Autodesk Inventor part; units mm, degrees
ref_plane "YZ Plane" through (0, 0, 0) normal (1, 0, 0) x (0, 1, 0)
ref_plane "XZ Plane" through (0, 0, 0) normal (0, 1, 0) x (-1, 0, 0)
ref_plane "XY Plane" through (0, 0, 0) normal (0, 0, 1) x (1, 0, 0)
sketch "Sketch1" plane through (0, 0, 0) normal (0, 1, 0) x (-1, 0, 0)
  line L0 (-35, 35) -> (35, 35)
  line L1 (35, 35) -> (35, -35)
  line L2 (35, -35) -> (-35, -35)
  line L3 (-35, -35) -> (-35, 35)
  line L4 (-35, 35) -> (35, -35) construction
  line L5 (35, 35) -> (-35, -35) construction
  point P0 (0, 0)
  dimension "d0" = 70
  dimension "d1" = 70
extrude "Extrusion1" add sketch "Sketch1" along normal blind 1
sketch "Sketch2" plane through (0, 1, 0) normal (0, 1, 0) x (1, 0, 0)
  line L0 (-17, -17) -> (-17, 35) construction
  line L1 (25, -35) -> (25, 35) construction
  line L2 (35, -35) -> (35, 35)
  line L3 (-35, 35) -> (-35, -35)
  line L4 (-10.2536, 14.5438) -> (28, -4.9295)
  line L5 (28, -4.9295) -> (28, -11.3476)
  line L6 (28, -11.3476) -> (-11.7123, 9.2196)
  line L7 (-11.7123, 9.2196) -> (-11.7123, -14.0097)
  line L8 (-11.7123, -14.0097) -> (-17, -14.0097)
  line L9 (-17, -14.0097) -> (-17, 14.5438)
  line L10 (-17, 14.5438) -> (-10.2536, 14.5438)
  point P0 (0, 0)
  dimension "d4" = 10
  dimension "d5" = 18
sketch "Sketch5" plane through (0, 1, 0) normal (0, 1, 0) x (1, 0, 0)
  circle A0 centre (-27, 0) radius 3.1
  line L0 (-35, 35) -> (-35, -35)
  line L1 (-35, 0) -> (0, 0) construction
  dimension "d14" = 6.2
  dimension "d15" = 8
extrude "Extrusion4" cut sketch "Sketch5" against normal up to next
fillet "Fillet1" radius 2 4 edges at (-35, 0.5, -35) (-35, 0.5, 35) (35, 0.5, -35) (35, 0.5, 35)
emboss "Emboss2" sketch "Sketch2" operation cut depth 0.1 direction (0, -1, 0)
properties part number "AntennaNameplate"
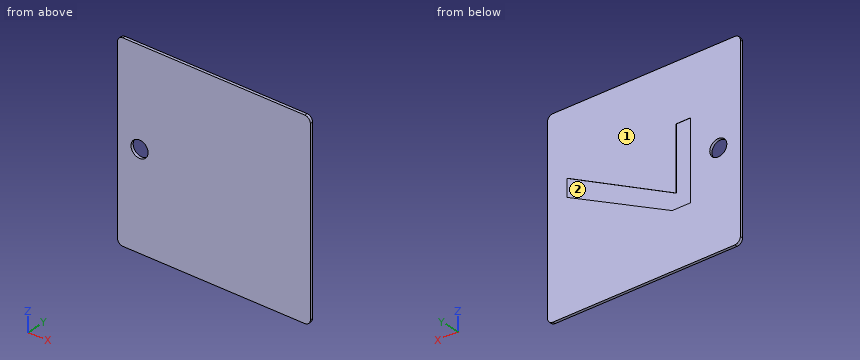
Check sheet for the modelled part. Datum: model origin and axes. Units: mm. Face numbers are marked on the shaded views. Round coordinates to 2 decimals unless told otherwise and drop trailing zeros. Loops run counter-clockwise (first coordinate to the right, second up) from the corner with the lowest first, then second, coordinate; pieces in that order, holes last. Notation, with made-up numbers: (83.25, 38.5) -> (120.25, 38.5) arc R23 cw to (120.25, 67.5) -> close; hole circle Ø7 at (47.5, 64.25). An arc over 180 degrees is marked (long way). Put each result on its own line as item: value. Start each with the question number.
1. Scan lines: probe 1 along Z at (x, y) = (-27, 0.6); probe 2 along X at (y, z) = (0.7, 0); probe 3 along X at (y, z) = (0.2, -2). Record each from-to range of solid material in increasing order.
2. Section check B-B (z = 0). Enter the section's corners in (x, y), plus the area to 3 significant figures.
3. Section check A-A (x = -27). Enter the section's corners in (y, z), plus the area to 3 significant figures.
4. Gauge pin test, flat end, axial feed: pin 1 (3.5 mm diameter, centred on x = -27, z = 0, fed in from -Y). Record the tip position at first contact, or that the pin passes through.
5. Draft check along X on the marked faces 1 and 2. Enter one of: +X half, -X half, draft (parallel to the pull), parting line (faces both ways), or undercut.
Findings:
1. probe 1: z = -35 to -3.1, 3.1 to 35
1. probe 2: x = -35 to -30.1, -23.9 to 35
1. probe 3: x = -35 to -29.37, -24.63 to 35
2. outline: (-35, 0) -> (-30.1, 0) -> (-30.1, 1) -> (-35, 1) -> close; (-23.9, 0) -> (35, 0) -> (35, 1) -> (18.32, 1) -> (18.32, 0.9) -> (6.09, 0.9) -> (6.09, 1) -> (-11.71, 1) -> (-11.71, 0.9) -> (-17, 0.9) -> (-17, 1) -> (-23.9, 1) -> close
2. area: 62.0 mm^2
3. outline: (0, -35) -> (1, -35) -> (1, -3.1) -> (0, -3.1) -> close; (0, 3.1) -> (1, 3.1) -> (1, 35) -> (0, 35) -> close
3. area: 63.8 mm^2
4. pin 1: passes through
5. face 1: draft
5. face 2: undercut
